For this review, take the finished solid that the model builds, in its own axes (mm). Round coordinates to 2 decimals unless told otherwise and drop trailing zeros. Write each loop counter-clockwise with the first axis right and the second up, starting at its lowest first coordinate (ties: lowest second). Pieces come first, ordered by that corner, then holes. Notation, with made-up numbers: (-31, 25.25) -> (-22, 25.25) arc R10 cw to (-22, 29.25) -> close; hole circle Ø1 at (34.25, 26.25). An arc over 180 degrees is marked (long way). Answer as CSV lines item,"result". Start each with the question number.
Item 1: For pin 1 Ø1 at (x, y) = (-1, -0.5) entering from -Z; pin 2 Ø0.9 at (x, z) = (-1.5, 2) entering from +Y; pin 3 Ø0.6 at (y, z) = (-1, 2) entering from -X, all flat-tipped, find the tip position at first contact; note any pin that passes through.
Item 2: Wall thickness on probe 1 along X at (y, z) = (-0.2, 11); probe 2 along X at (y, z) = (0, 5.25): over which ranges is each line inside the solid? List them lowest first. Write a range as from..to.
Item 3: Take a section at A-A on z = 10.75. Give the boundary of the cut face in (x, y).
Item 4: Take a section at C-C on y = -0.95. Give the boundary of the cut face in (x, z).
Item 5: Take a section at B-B on x = -1.2. Give the boundary of the cut face in (y, z).
```python
from build123d import *

# Parameters (mm, degrees)
F3_DEPTH = 0.2
F4_COUNT = 4


# Not quite as in the source:
# - a feature names something its author has since deleted; it is built from what else it names


with BuildPart() as f1:
    # F0 (on Front) → F1 (revolve)
    with BuildSketch(Plane.XZ):
        with BuildLine():
            Line((0, 20.1388888889), (0, 0))
            Line((0, 0), (0.5208333333, 0))
            ThreePointArc((0.5208333333, 0), (0.5624944489, 0.6938891109), (0.5763888889, 1.3888888889))
            Line((0.5763888889, 1.3888888889), (0.5763888889, 17.8472222222))
            ThreePointArc((0.5763888889, 17.8472222222), (0.5492348486, 18.7862912781), (0.467863469, 19.7222222222))
            ThreePointArc((0.467863469, 19.7222222222), (0.3132520298, 20.01962212), (0, 20.1388888889))
        make_face()
    revolve(axis=Axis((0, 0, 10.0694444444), (0, 0, 1)))

    # F2 (on Front) → F3 (join, symmetric)
    with BuildSketch(Plane.XZ):
        Polygon((0, 11.1135402694), (0, 1.4373737374), (1.9097222222, 1.5068181818), (1.9097222222, 1.854040404), (0.4, 2.2865129156), (0.4, 11.3888888889), align=None)
    extrude(amount=F3_DEPTH, both=True)

    # F4: F1 ×4 about axis
    f4_axis = Axis((0, 0, 1.3888888889), (0, 0, 1))


with BuildPart() as f1_1:
    add(f1.part)
    for i in range(1, F4_COUNT):
        add(f1.part.rotate(f4_axis, i * 360 / F4_COUNT))


solid = f1_1.part
```
Output values:
1,pin 1,"stops at z = 1.46"
1,pin 2,"stops at y = 0.2"
1,pin 3,"stops at x = -0.2"
2,probe 1,"x = -0.54..0.54"
2,probe 2,"x = -0.58..0.58"
3,outline,"circle Ø1.15 at (0, 0)"
4,outline,"(-0.2, 1.47) -> (0.2, 1.47) -> (0.2, 2.13) -> (-0.2, 2.13) -> close"
5,outline,"(-0.2, 1.48) -> (0.2, 1.48) -> (0.2, 2.06) -> (-0.2, 2.06) -> close"
